from build123d import *

# Parameters (mm, degrees)
RESSALTO_EXTRUS_O1_DEPTH   = 250
ESCALA1_SCALE              = 1.5
CORTE_EXTRUS_O1_START      = -75
CORTE_EXTRUS_O1_DEPTH      = 225
CORTE_EXTRUS_O3_DEPTH      = 344.667466727
CORTE_EXTRUS_O3_DEPTH_BACK = 344.667466727
ESBO_O7_R                  = 36
CORTE_EXTRUS_O4_DEPTH      = 69
ESBO_O7_3_R                = 30
CORTE_EXTRUS_O5_DEPTH      = 395.013784799
CORTE_EXTRUS_O6_START      = -306
ESBO_O7_4_R                = 36
ESBO_O7_4_R_2              = 30
CORTE_EXTRUS_O6_DEPTH      = 69


with BuildPart() as part:
    # Esboço1 → Ressalto-extrusão1 (new body)
    with BuildSketch(Plane.XY):
        with BuildLine():
            Line((65, 0), (64.021024633, -14))
            Line((64.021024633, -14), (56.886629039, -33.601590794))
            Line((56.886629039, -33.601590794), (-36.113370961, -50))
            Line((-36.113370961, -50), (-47.32844057, -45.918048487))
            Line((-47.32844057, -45.918048487), (-55, -36.775439975))
            Line((-55, -36.775439975), (-55, 9.746573698))
            Line((-55, 9.746573698), (-47, 20.366669268))
            Line((-47, 20.366669268), (-36.113370961, 28))
            Line((-36.113370961, 28), (27, 20))
            Line((27, 20), (32.013345877, 9.746573698))
            ThreePointArc((32.013345877, 9.746573698), (40.293006212, 1.034435734), (52.07121536, -1.358870022))
            Line((52.07121536, -1.358870022), (65, 0))
        make_face()
    extrude(amount=RESSALTO_EXTRUS_O1_DEPTH)


with BuildPart() as part_1:
    # Escala1: scaled about (-3.384050485, -11.684350271, 125)
    add(part.part.scale(ESCALA1_SCALE).moved(Location((1.692025242, 5.842175135, -62.5))))

    # Esboço4 → Corte-extrusão1 (cut)
    with BuildSketch(Plane(origin=(0, 0, -62.5), x_dir=(-1, 0, 0), z_dir=(0, 0, -1)).offset(CORTE_EXTRUS_O1_START)):
        Polygon((69.300635612, -63.034897595), (80.807974757, -49.320984827), (-87.021968802, -44.560211056), (52.478031198, -69.157824864), align=None)
        Polygon((-42.192025243, 35.842175136), (80.807974757, 20.462035682), (68.807974757, 36.392179037), (52.478031198, 47.842175136), align=None)
    extrude(amount=-CORTE_EXTRUS_O1_DEPTH, mode=Mode.SUBTRACT)

    # Esboço6 → Corte-extrusão3 (cut, two sides: drawn at the far end of the back side and taken through both)
    with BuildSketch(Plane(origin=(-3.763238402, 30.095846977, 0), x_dir=(0.9922727729449546, 0.12407555791585548, 0), z_dir=(-0.12407555791585548, 0.9922727729449546, 0)).offset(-CORTE_EXTRUS_O3_DEPTH_BACK)):
        with BuildLine():
            Line((-27.644714695, -37.5), (-3.68686424, -37.5))
            ThreePointArc((-3.68686424, -37.5), (13.99080529, -44.82233047), (21.31313576, -62.5))
            Line((21.31313576, -62.5), (21.31313576, -187.5))
            ThreePointArc((21.31313576, -187.5), (13.99080529, -205.17766953), (-3.68686424, -212.5))
            Line((-3.68686424, -212.5), (-27.644714695, -212.5))
            ThreePointArc((-27.644714695, -212.5), (-45.322384225, -205.17766953), (-52.644714695, -187.5))
            Line((-52.644714695, -187.5), (-52.644714695, -62.5))
            ThreePointArc((-52.644714695, -62.5), (-45.322384225, -44.82233047), (-27.644714695, -37.5))
        make_face()
    extrude(amount=CORTE_EXTRUS_O3_DEPTH + CORTE_EXTRUS_O3_DEPTH_BACK, mode=Mode.SUBTRACT)

    # Esboço7 → Corte-extrusão4 (cut)
    with BuildSketch(Plane.XY.offset(312.5)):
        with Locations((2.82595792, -11.797691618)):
            Circle(ESBO_O7_R)
    extrude(amount=-CORTE_EXTRUS_O4_DEPTH, mode=Mode.SUBTRACT)

    # Esboço7<3> → Corte-extrusão5 (cut, through all)
    with BuildSketch(Plane.XY.offset(312.5)):
        with Locations((2.82595792, -11.797691618)):
            Circle(ESBO_O7_3_R)
    extrude(amount=-CORTE_EXTRUS_O5_DEPTH, mode=Mode.SUBTRACT)

    # Esboço7<4> → Corte-extrusão6 (cut)
    with BuildSketch(Plane.XY.offset(312.5).offset(CORTE_EXTRUS_O6_START)):
        with Locations((2.82595792, -11.797691618)):
            Circle(ESBO_O7_4_R)
        with Locations((2.82595792, -11.797691618)):
            Circle(ESBO_O7_4_R_2, mode=Mode.SUBTRACT)
    extrude(amount=-CORTE_EXTRUS_O6_DEPTH, mode=Mode.SUBTRACT)


solid = part_1.part
Check sheet for the modelled part. Datum: model origin and axes. Units: mm. A direction names the side the tool comes from. Coordinates: 2 decimals unless noted, no trailing zeros. Loops run counter-clockwise (first coordinate to the right, second up) from the corner with the lowest first, then second, coordinate; pieces in that order, holes last. Notation, with made-up numbers: (-12, 56.5) -> (6, 56.5) arc R32 cw to (6, 93.5) -> close; hole circle Ø7 at (-8, 4.25). An arc over 180 degrees is marked (long way). Write item = value, one per line. Start each with the question number.
1. Depth check by flat-ended pin: P1, Ø8, axis at x = -11.5, z = 236.5, coming from the -Y side; P2, Ø12.5, axis at x = -18.5, y = 6.5, coming from the +Z side; P3, Ø1.5, axis at y = 7, z = 62.5, coming from the +X side. Enter the tip coordinate at first touch or a pass-through.
2. Material ranges on line 1 (Z direction, x = -57.5, y = 36); line 2 (X direction, y = -32, z = 285); line 3 (Z direction, x = -20, y = 19), recorded low to high.
3. Draft check along X on faces 5 (the flat face through (-30, -36, 312.5)), 6 (the cylindrical face through (22.23, -41.17, 201.61)), 7 (the flat face through (-60.757, 42.037, 274.475)). Enter one of: released by +X, released by -X, zero draft, split by the parting line, or undercut.
4. Tool access check on faces 1 (the cylindrical face through (19.438, -43.736, -27.517)), 2 (the flat face through (-59.447, 23.133, 123.425)), 3 (the cylindrical face through (-44.2, -13.2, 45)), 4 (the flat face through (18.643, 22.677, 124.125)). Record the directions out of +Z, -Z, +X, -X, +Y, -Y that give a thin tool (end or side, any length) a straight path to the whole face; none if there is none.
5. Section check A-A on x = -14. Give the number of separate pieces and of enclosed holes in the cut face, then the cut area to 3 significant figures.
6. Section check B-B on z = 81. Record the cut outline in (x, y), then the cut area to 3 significant figures.
7. Section check D-D on x = 69. Record the cut outline in (y, z).
8. Section check C-C on z = -15.5. Record the cut outline in (x, y).
Responses:
q1.P1 = -62.62
q1.P2 = 243.5
q1.P3 = 64.42
q2.line_1 = -62.5 to 12.5, 237.5 to 312.5
q2.line_2 = -80.81 to -26.97, 32.62 to 91.59
q2.line_3 = -62.5 to 37.5, 212.5 to 312.5
q3.face_5 = zero draft
q3.face_6 = undercut
q3.face_7 = released by -X
q4.face_1 = -Z
q4.face_2 = -X, +Y
q4.face_3 = +Y
q4.face_4 = -Y
q5.separate_pieces = 4
q5.enclosed_holes = 0
q5.area = 7,750 mm2
q6.outline = (-80.81, -49.32) -> (-47.01, -48.36) -> (-56, 23.56) -> (-80.81, 20.46) -> close; (17.39, 32.74) -> (19.87, 12.89) arc R30 cw to (25.42, -31.53) -> (27.26, -46.26) -> (87.02, -44.56) -> (97.72, -15.16) -> (99.19, 5.84) -> (79.8, 3.8) arc R30 cw to (49.71, 20.46) -> (42.19, 35.84) -> close
q6.area = 6,280 mm2
q7.outline = (-47.74, -62.5) -> (4.63, -62.5) -> (4.63, 312.5) -> (-47.74, 312.5) -> (-47.74, 237.5) -> (-45.07, 237.5) -> (-45.07, 12.5) -> (-47.74, 12.5) -> close
q8.outline = (-80.81, -49.32) -> (-69.3, -63.03) -> (-52.48, -69.16) -> (87.02, -44.56) -> (97.72, -15.16) -> (99.19, 5.84) -> (79.8, 3.8) arc R30 cw to (49.71, 20.46) -> (42.19, 35.84) -> (-52.48, 47.84) -> (-68.81, 36.39) -> (-80.81, 20.46) -> close; hole circle Ø72 at (2.83, -11.8)
